The model under review builds one solid part; all positions refer to its coordinate system, in mm. Round coordinates to 2 decimals unless told otherwise and drop trailing zeros. Write each loop counter-clockwise with the first axis right and the second up, starting at its lowest first coordinate (ties: lowest second). Pieces come first, ordered by that corner, then holes. Notation, with made-up numbers: (51.25, 9.25) -> (81.25, 9.25) arc R25 ccw to (81.25, 38.25) -> close; hole circle Ø4 at (-13.5, 18.5). An arc over 180 degrees is marked (long way). Use CSV: the item, a comma, the result in double quotes. Start each with the question number.
1) For pin 1 Ø5 at (y, z) = (-1379, 9) entering from -X; pin 2 Ø1 at (y, z) = (-1238.5, 4) entering from +X, all flat-tipped, find the tip position at first contact; note any pin that passes through.
2) Take a section at A-A, the plane z = 11.75. Give the boundary of the cut face in (x, y).
3) Wall thickness on probe 1 along Y at (x, z) = (9147.5, 24); probe 2 along X at (y, z) = (-1392.5, 9); probe 3 along Y at (x, z) = (9734.5, 5.5): over which ranges is each line inside the solid? List them lowest first. Write a range as [from, to].
4) Take a section at B-B, the plane y = -1182. Give the boundary of the cut face in (x, z).
5) Take a section at C-C, the plane x = 8600.5. Give the boundary of the cut face in (y, z).
from build123d import *

# Parameters (mm, degrees)
F1_DEPTH = 1
F2_DEPTH = 25


# Not quite as in the source:
# - a feature names something its author has since deleted; it is built from what else it names


with BuildPart() as f1:
    # F0 (on Top) → F1 (new body)
    with BuildSketch(Plane.XY):
        with BuildLine():
            Line((9646.8274642131, -957.7307995355), (8146.8274642131, -957.7307995355))
            Line((8146.8274642131, -957.7307995355), (7830.554096613, -1573.7270701518))
            ThreePointArc((7830.554096613, -1573.7270701518), (7832.0390367178, -1759.2626053639), (7985.3704990637, -1863.7379734104))
            Line((7985.3704990637, -1863.7379734104), (8329.6804291381, -1903.7785528549))
            ThreePointArc((8329.6804291381, -1903.7785528549), (8413.0435068902, -1933.1322385833), (8475.616358081, -1995.5476204376))
            Line((8475.616358081, -1995.5476204376), (8744.9993562468, -2421.5486497246))
            ThreePointArc((8744.9993562468, -2421.5486497246), (9097.0590224145, -2649.3179001076), (9498.727349417, -2528.9543049258))
            Line((9498.727349417, -2528.9543049258), (10081.2209659321, -2014.102836222))
            ThreePointArc((10081.2209659321, -2014.102836222), (10146.2998029037, -1895.5752337571), (10121.0868255742, -1762.7281286256))
            Line((10121.0868255742, -1762.7281286256), (9646.8274642131, -957.7307995355))
        make_face()
    extrude(amount=F1_DEPTH)

    # F0 (on Top) → F2 (join)
    with BuildSketch(Plane.XY):
        with BuildLine():
            Line((9646.8274642131, -957.7307995355), (8146.8274642131, -957.7307995355))
            Line((8146.8274642131, -957.7307995355), (7830.554096613, -1573.7270701518))
            ThreePointArc((7830.554096613, -1573.7270701518), (7832.0390367178, -1759.2626053639), (7985.3704990637, -1863.7379734104))
            Line((7985.3704990637, -1863.7379734104), (8329.6804291381, -1903.7785528549))
            ThreePointArc((8329.6804291381, -1903.7785528549), (8413.0435068902, -1933.1322385833), (8475.616358081, -1995.5476204376))
            Line((8475.616358081, -1995.5476204376), (8744.9993562468, -2421.5486497246))
            ThreePointArc((8744.9993562468, -2421.5486497246), (9097.0590224145, -2649.3179001076), (9498.727349417, -2528.9543049258))
            Line((9498.727349417, -2528.9543049258), (10081.2209659321, -2014.102836222))
            ThreePointArc((10081.2209659321, -2014.102836222), (10146.2998029037, -1895.5752337571), (10121.0868255742, -1762.7281286256))
            Line((10121.0868255742, -1762.7281286256), (9646.8274642131, -957.7307995355))
        make_face()
    extrude(amount=F2_DEPTH)


solid = f1.part
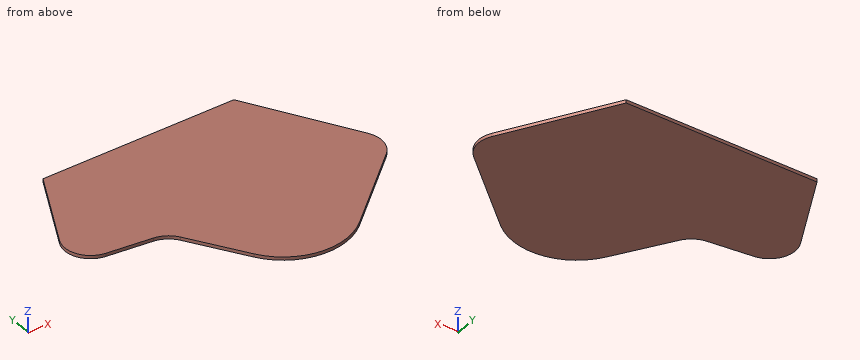
Values found:
1,pin 1,"x = 7929.25"
1,pin 2,"x = 9812.54"
2,outline,"(7830.55, -1573.73) arc R200 ccw to (7985.37, -1863.74) -> (8329.68, -1903.78) arc R200 cw to (8475.62, -1995.55) -> (8745, -2421.55) arc R500 ccw to (9498.73, -2528.95) -> (10081.22, -2014.1) arc R200 ccw to (10121.09, -1762.73) -> (9646.83, -957.73) -> (8146.83, -957.73) -> close"
3,probe 1,"[-2653.91, -957.73]"
3,probe 2,"[7923.6, 9902.97]"
3,probe 3,"[-2320.56, -1106.54]"
4,outline,"(8031.68, 0) -> (9778.95, 0) -> (9778.95, 25) -> (8031.68, 25) -> close"
5,outline,"(-2193.04, 0) -> (-957.73, 0) -> (-957.73, 25) -> (-2193.04, 25) -> close"
